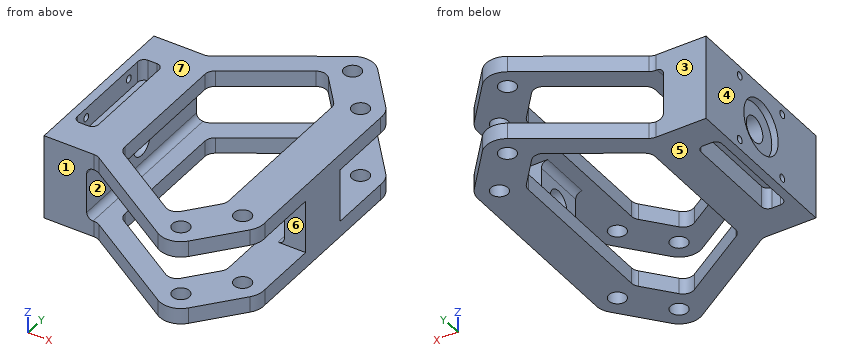
from build123d import *

# Parameters (mm, degrees)
SKETCH1_R               = 4
BOSS_EXTRUDE1_DEPTH     = 40
SKETCH2_W               = 100
SKETCH2_H               = 25
CUT_EXTRUDE1_DEPTH      = 113.5
CUT_EXTRUDE1_DEPTH_BACK = 33.5
SKETCH3_W               = 25
SKETCH3_H               = 25
BOSS_EXTRUDE2_DEPTH     = 10
SKETCH4_R               = 6
CUT_EXTRUDE2_DEPTH      = 100
FILLET1_R               = 5
FILLET2_R               = 3
SKETCH5_R               = 1.75
CUT_EXTRUDE3_DEPTH      = 10
SKETCH7_W               = 10
SKETCH7_H               = 50
CUT_EXTRUDE4_DEPTH      = 10
FILLET3_R               = 3
FILLET3_OF_MIRROR1_R    = 3
SKETCH8_R               = 12.5
CUT_EXTRUDE5_DEPTH      = 3


with BuildPart() as part:
    # Sketch1 → Boss-Extrude1 (new body)
    with BuildSketch(Plane.XY):
        with BuildLine():
            Line((25, 0), (73.308886978, -30.922345302))
            ThreePointArc((73.308886978, -30.922345302), (80.218691228, -32.384006119), (86.370944241, -28.915342115))
            Line((86.370944241, -28.915342115), (102.720944241, -9.365342115))
            ThreePointArc((102.720944241, -9.365342115), (104.608588105, -5.888263678), (105, -1.951250782))
            Line((105, -1.951250782), (105, 0))
            Line((105, 0), (105, 80))
            Line((105, 80), (105, 81.951250782))
            ThreePointArc((105, 81.951250782), (104.608588105, 85.888263678), (102.720944241, 89.365342115))
            Line((102.720944241, 89.365342115), (86.370944241, 108.915342115))
            ThreePointArc((86.370944241, 108.915342115), (80.218691228, 112.384006119), (73.308886978, 110.922345302))
            Line((73.308886978, 110.922345302), (25, 80))
            Line((25, 80), (0, 80))
            Line((0, 80), (0, 0))
            Line((0, 0), (25, 0))
        make_face()
        with Locations((78.7, -22.5)):
            Circle(SKETCH1_R, mode=Mode.SUBTRACT)
        with Locations((95.05, -2.95)):
            Circle(SKETCH1_R, mode=Mode.SUBTRACT)
        with Locations((78.7, 102.5)):
            Circle(SKETCH1_R, mode=Mode.SUBTRACT)
        with Locations((95.05, 82.95)):
            Circle(SKETCH1_R, mode=Mode.SUBTRACT)
        Polygon((30.852797713, 71.873177413), (30.852797713, 8.126822587), (70.209148437, -17.065036365), (85, 0.620660764), (85, 79.379339236), (70.209148437, 97.065036365), align=None, mode=Mode.SUBTRACT)
    extrude(amount=-BOSS_EXTRUDE1_DEPTH)

    # Sketch2 → Cut-Extrude1 (cut, two sides)
    with BuildSketch(Plane(origin=(0, 0, 0), x_dir=(1, 0, 0), z_dir=(0, 1, 0))) as cut_extrude1_sk:
        with Locations((70, 20)):
            Rectangle(SKETCH2_W, SKETCH2_H)
    extrude(amount=CUT_EXTRUDE1_DEPTH, mode=Mode.SUBTRACT)
    extrude(cut_extrude1_sk.sketch, amount=-CUT_EXTRUDE1_DEPTH_BACK, mode=Mode.SUBTRACT)

    # Sketch3 → Boss-Extrude2 (add)
    with BuildSketch(Plane(origin=(105, 0, 0), x_dir=(0, 0, -1), z_dir=(1, 0, 0))):
        with Locations((20, 40)):
            Rectangle(SKETCH3_W, SKETCH3_H)
    extrude(amount=-BOSS_EXTRUDE2_DEPTH)

    # Sketch4 → Cut-Extrude2 (cut)
    with BuildSketch(Plane.ZY):
        with Locations((-20, 40)):
            Circle(SKETCH4_R)
    extrude(amount=-CUT_EXTRUDE2_DEPTH, mode=Mode.SUBTRACT)

    # Fillet1
    fillet1_edges = [part.edges().sort_by_distance(p)[0] for p in [
        (25, 80, -3.75),
        (25, 80, -36.25),
        (25, 0, -36.25),
        (85, 79.379339236, -36.25),
        (85, 0.620660764, -36.25),
        (70.209148437, -17.065036365, -36.25),
        (30.852797713, 8.126822587, -36.25),
        (30.852797713, 71.873177413, -36.25),
        (70.209148437, 97.065036365, -36.25),
        (70.209148437, 97.065036365, -3.75),
        (85, 79.379339236, -3.75),
        (30.852797713, 71.873177413, -3.75),
        (30.852797713, 8.126822587, -3.75),
        (70.209148437, -17.065036365, -3.75),
        (85, 0.620660764, -3.75),
        (25, 0, -3.75),
    ]]
    fillet(fillet1_edges, radius=FILLET1_R)

    # Fillet2
    fillet2_edges = [part.edges().sort_by_distance(p)[0] for p in [
        (20, 40, -32.5),
        (20, 40, -7.5),
        (95, 40, -32.5),
        (95, 40, -7.5),
    ]]
    fillet(fillet2_edges, radius=FILLET2_R)

    # Sketch5 → Cut-Extrude3 (cut)
    with BuildSketch(Plane.ZY):
        with Locations((-35.5, 55.5)):
            Circle(SKETCH5_R)
        with Locations((-4.5, 55.5)):
            Circle(SKETCH5_R)
        with Locations((-35.5, 24.5)):
            Circle(SKETCH5_R)
        with Locations((-4.5, 24.5)):
            Circle(SKETCH5_R)
    extrude(amount=-CUT_EXTRUDE3_DEPTH, mode=Mode.SUBTRACT)

    # Sketch7 → Cut-Extrude4 (cut)
    with BuildSketch(Plane.XY):
        with Locations((9, 40)):
            Rectangle(SKETCH7_W, SKETCH7_H)
    cut_extrude4 = extrude(amount=-CUT_EXTRUDE4_DEPTH, mode=Mode.SUBTRACT)

    # Fillet3
    fillet3_edges = [part.edges().sort_by_distance(p)[0] for p in [
        (4, 15, -5),
        (4, 65, -5),
        (14, 65, -5),
        (14, 15, -5),
    ]]
    fillet(fillet3_edges, radius=FILLET3_R)

    # Mirror1: Cut-Extrude4 across plane
    add(cut_extrude4.mirror(Plane.XY.offset(-20)), mode=Mode.SUBTRACT)

    # Fillet3 of Mirror1
    fillet3_of_mirror1_edges = [part.edges().sort_by_distance(p)[0] for p in [
        (4, 15, -35),
        (4, 65, -35),
        (14, 65, -35),
        (14, 15, -35),
    ]]
    fillet(fillet3_of_mirror1_edges, radius=FILLET3_OF_MIRROR1_R)

    # Sketch8 → Cut-Extrude5 (cut)
    with BuildSketch(Plane.ZY):
        with Locations((-20, 40)):
            Circle(SKETCH8_R)
    extrude(amount=-CUT_EXTRUDE5_DEPTH, mode=Mode.SUBTRACT)


solid = part.part
Could you check a few things on this model? Use its own coordinates, in mm. Face numbers are marked on the shaded views. A direction names the side the tool comes from. Give positions to 0.01 mm unless a question says otherwise; leave off trailing zeros. Write each loop counter-clockwise with the first axis right and the second up, starting at its lowest first coordinate (ties: lowest second). Pieces come first, ordered by that corner, then holes. Notation, with made-up numbers: (25, 78) -> (56, 78) arc R6 cw to (56, 83) -> close; hole circle Ø2 at (-20, 7.5). An arc over 180 degrees is marked (long way). Answer as a JSON object with one key per item and string values.
Q1. Suppose I cut it at B-B on z = -20. Write out the boundary of the cut face in (x, y).
Taken from the geometry:
{"outline": "(0, 0) -> (20, 0) -> (20, 34) -> (3, 34) -> (3, 27.5) -> (0, 27.5) -> close; (0, 52.5) -> (3, 52.5) -> (3, 46) -> (20, 46) -> (20, 80) -> (0, 80) -> close; (95, 27.5) -> (105, 27.5) -> (105, 52.5) -> (95, 52.5) -> (95, 46) -> (100, 46) -> (100, 34) -> (95, 34) -> close"}
Q2. Please list where these lines run through material, in increasing order: L1, parallel to X at y = 31, z = -38; L2, parallel to Y at x = 2, z = -35.5; L3, parallel to Y at x = 78.7, z = -35.5.
Taken from the geometry:
{"L1": "x = 0 to 4, 14 to 30.85, 85 to 105", "L2": "y = 0 to 22.75, 26.25 to 53.75, 57.25 to 80", "L3": "y = -32.5 to -26.5, -18.5 to -6.91, 86.91 to 98.5, 106.5 to 112.5"}
Q3. We'd pull the mould along Z, two halves only. Please class the marked faces 4, 5, 6 and 7: released by +Z, released by -Z, zero draft, split by the parting line, or undercut.
Taken from the geometry:
{"face 4": "zero draft", "face 5": "released by -Z", "face 6": "undercut", "face 7": "released by +Z"}
Q4. Suppose I cut it at D-D on x = 46. Write out the boundary of the cut face in (y, z).
Taken from the geometry:
{"outline": "(-13.44, -40) -> (-1.57, -40) -> (-1.57, -32.5) -> (-13.44, -32.5) -> close; (-13.44, -7.5) -> (-1.57, -7.5) -> (-1.57, 0) -> (-13.44, 0) -> close; (81.57, -40) -> (93.44, -40) -> (93.44, -32.5) -> (81.57, -32.5) -> close; (81.57, -7.5) -> (93.44, -7.5) -> (93.44, 0) -> (81.57, 0) -> close"}
Q5. Will these pins go through, and if not, where does the flat tip stop? pin 1 Ø14.5 at (x, z) = (97, -24) entering from +Y; pin 2 Ø3 at (x, z) = (9.5, -5.5) entering from +Y; pin 3 Ø21 at (y, z) = (45, -18.5) entering from +X; pin 4 Ø10 at (x, z) = (57, -16) entering from -Y.
Taken from the geometry:
{"pin 1": "stops at y = 52.5", "pin 2": "stops at y = 80", "pin 3": "stops at x = 105", "pin 4": "passes through"}
Q6. Suppose I cut it at C-C on y = 5. Write out the boundary of the cut face in (x, z), then the cut area to 3 significant figures.
Taken from the geometry:
{"outline": "(0, -40) -> (35.74, -40) -> (35.74, -32.5) -> (23, -32.5) arc R3 cw to (20, -29.5) -> (20, -10.5) arc R3 cw to (23, -7.5) -> (35.74, -7.5) -> (35.74, 0) -> (0, 0) -> close; (85, -40) -> (105, -40) -> (105, -32.5) -> (85, -32.5) -> close; (85, -7.5) -> (105, -7.5) -> (105, 0) -> (85, 0) -> close", "area": "1,340 mm²"}
Q7. Which directions (+Z, -Z, +X, -X, +Y, -Y) give clear straight access to the entire face, cutting with the end or side of a thin tool? Please do the marked faces 1, 2 and 3.
Taken from the geometry:
{"face 1": "+Z, -Z, -X, -Y", "face 2": "+Y, -Y", "face 3": "+Z, -Z, -X, +Y"}
